Here's how the part is built. I have some questions about the finished solid (model axes, mm). Round coordinates to 2 decimals unless told otherwise and drop trailing zeros. Order: outer loops, then holes, each group sorted by start corner. A loop starts at its lowest first (then second) coordinate and runs counter-clockwise, first axis right, second up. Notation, with made-up numbers: (31, 72) - (57, 72) arc R19 cw to (57, 106) - close; hole circle Ø6 at (31, 26.5). An arc over 180 degrees is marked (long way). Answer as a JSON object with one key per item and string values.
Autodesk Fusion 360 part; units mm, degrees
sketch "Boceto1" plane through (0, 0, 0) normal (0, 0, 1) x (1, 0, 0)
  spline S0 degree 5 poles (17, 50) (17.32, 49.4691) (17.96, 48.4536) (18.92, 47.0694) (20.2, 45.5067) (21.8, 44.0566) (23.4, 43.1548) (25, 42.846) (26.6, 43.1548) (28.2, 44.0566) (29.8, 45.5067) (31.08, 47.0694) (32.04, 48.4536) (32.68, 49.4691) (33, 50) knots 0 0 0 0 0 0 0.1 0.2 0.3 0.4 0.5 0.6 0.7 0.8 0.9 1 1 1 1 1 1
  line L0 (25, 43) -> (25, 0) construction
  arc A0 (7, 45) -> (17, 50) centre (4.4264, 62.6472) ccw
  arc A1 (0, 33) -> (7, 45) centre (-11.8333, 47.9444) ccw
  arc A2 (8.6345, 29.0047) -> (0, 33) centre (-8.4336, 3.4454) ccw
  line L1 (8.6345, 29.0047) -> (11.4903, 32.3049)
  arc A3 (11.4903, 0) -> (11.4903, 32.3049) centre (-162.0039, 16.1524) ccw
  arc A4 (33, 50) -> (43, 45) centre (45.5736, 62.6472) ccw
  arc A5 (43, 45) -> (50, 33) centre (61.8333, 47.9444) ccw
  arc A6 (50, 33) -> (41.3655, 29.0047) centre (58.4336, 3.4454) ccw
  line L2 (41.3655, 29.0047) -> (38.5097, 32.3049)
  arc A7 (38.5097, 32.3049) -> (38.5097, 0) centre (212.0039, 16.1524) ccw
  line L3 (17, 50) -> (33, 50)
  circle A8 centre (25, 47) radius 1.5
  line L4 (18, 0) -> (15, 0)
  line L5 (19, 41) -> (19, 0)
  line L6 (19, 0) -> (15, 0)
  line L7 (15, 0) -> (15, 41)
  line L8 (23, 41) -> (23, 0)
  line L9 (23, 0) -> (27, 0)
  line L10 (27, 0) -> (27, 41)
  line L11 (31, 41) -> (31, 0)
  line L12 (31, 0) -> (35, 0)
  line L13 (35, 0) -> (35, 41)
  arc A9 (23, 41) -> (27, 41) centre (25, 44.75) ccw
  arc A10 (15, 41) -> (19, 41) centre (17, 44.75) ccw
  arc A11 (31, 41) -> (35, 41) centre (33, 44.75) ccw
  line L14 (11.4903, 0) -> (38.5097, 0)
  point P0 (25, 43)
  dimension "d10" = 3
  dimension "d11" = 4
  dimension "d12" = 4
  dimension "d15" = 4
  dimension "d16" = 4
  dimension "d17" = 4
  dimension "d18" = 174.2445
  dimension "d19" = 19.0621
  dimension "d20" = 30.7343
  dimension "d21" = 17.8339
  dimension "d22" = 4.25
  dimension "d23" = 2
  dimension "d24" = 1
  dimension "d25" = 8.4336
  dimension "d26" = 3.4454
  dimension "d27" = 33.4336
  dimension "d28" = 46.5546
  dimension "d29" = 43.5546
  dimension "d30" = 39.5546
  dimension "d31" = 40.871
  dimension "d32" = 220.4376
  dimension "d33" = 70.267
  dimension "d34" = 59.2018
  dimension "d35" = 49.7991
extrude "Extruir1" add sketch "Boceto1" along normal blind 2 contours S0 A0 A1 A2 L1 A3 A4 A5 A6 L2 A7 L5 L7 L8 L10 L11 L13 A9 A10 A11 L14
extrude "Extruir2" add sketch "Boceto1" along normal blind 3 contours L4 L5 L6 L7 A10 L14
extrude "Extruir3" add sketch "Boceto1" along normal blind 3 contours L8 L9 L10 A9 L14
extrude "Extruir4" add sketch "Boceto1" along normal blind 3 contours L11 L12 L13 A11 L14
extrude "Extruir5" add sketch "Boceto1" along normal blind 1.5 contours S0 L3
1. If I drill on L1, parallel to X at y = 24.5, z = 2.65; L2, parallel to Y at x = 25, z = 0.95; L3, parallel to Z at x = 22, y = 29.5, over which ranges is the centre line in solid material (lowest first)? Write a range as [from, to].
Responses:
{"L1": "[15, 19], [23, 27], [31, 35]", "L2": "[0, 45.5], [48.5, 50]", "L3": "[0, 2]"}
2. For P1, Ø3.5, axis at x = 25, y = 47, coming from the +Z side; P2, Ø5, axis at x = 30.5, y = 27.5, coming from the -Z side; P3, Ø1.1, axis at y = 22.5, z = 2.5, coming from the -X side; P4, Ø1.1, axis at y = 28.5, z = 2.5, coming from the +X side, each with a flat end and sliding along its axis, tell me the tip position at first contact or that it passes through.
Responses:
{"P1": "z = 1.5", "P2": "z = 0", "P3": "x = 12.12", "P4": "x = 38.21"}
3. Imagine slicing it at C-C (x = 46). List the corners of the cut face in (y, z) for me.
Responses:
{"outline": "(31.55, 0) - (37.33, 0) - (37.33, 2) - (31.55, 2) - close"}
4. Imagine slicing it at D-D (y = 22.5). List the corners of the cut face in (x, z) for me.
Responses:
{"outline": "(12.12, 0) - (37.88, 0) - (37.88, 2) - (35, 2) - (35, 3) - (31, 3) - (31, 2) - (27, 2) - (27, 3) - (23, 3) - (23, 2) - (19, 2) - (19, 3) - (15, 3) - (15, 2) - (12.12, 2) - close"}
5. Imagine slicing it at B-B (y = 15.5). List the corners of the cut face in (x, z) for me.
Responses:
{"outline": "(12.24, 0) - (37.76, 0) - (37.76, 2) - (35, 2) - (35, 3) - (31, 3) - (31, 2) - (27, 2) - (27, 3) - (23, 3) - (23, 2) - (19, 2) - (19, 3) - (15, 3) - (15, 2) - (12.24, 2) - close"}
6. Thinking about a two-plate mould opening in Y: for faces 1 (the face through (25, 50, 1)), 2 (the face through (45.47, 31.31, 0.99)), 3 (the face through (24.675, 48.464, 0.74)), 4 (the face through (25, 49, 1.5)), which applies, pulls with the +Y half, pulls with the -Y half, needs draft (parallel to the pull), parting line crosses it, or undercut?
Responses:
{"face 1": "pulls with the +Y half", "face 2": "pulls with the -Y half", "face 3": "undercut", "face 4": "needs draft"}
7. Imagine slicing it at A-A (z = 0.95). List the corners of the cut face in (x, y) for me.
Responses:
{"outline": "(0, 33) arc R30.73 cw to (8.63, 29) - (11.49, 32.3) arc R174.24 cw to (11.49, 0) - (38.51, 0) arc R174.24 cw to (38.51, 32.3) - (41.37, 29) arc R30.73 cw to (50, 33) arc R19.06 cw to (43, 45) arc R17.83 cw to (33, 50) - (17, 50) arc R17.83 cw to (7, 45) arc R19.06 cw to start; hole circle Ø3 at (25, 47)"}
